Read the model definition and answer for the solid it produces. Units are mm, in the model's axes. Face numbers are marked on the shaded views. A direction names the side the tool comes from. Give positions to 0.01 mm unless a question says otherwise; leave off trailing zeros. Write each loop counter-clockwise with the first axis right and the second up, starting at its lowest first coordinate (ties: lowest second). Pieces come first, ordered by that corner, then holes.
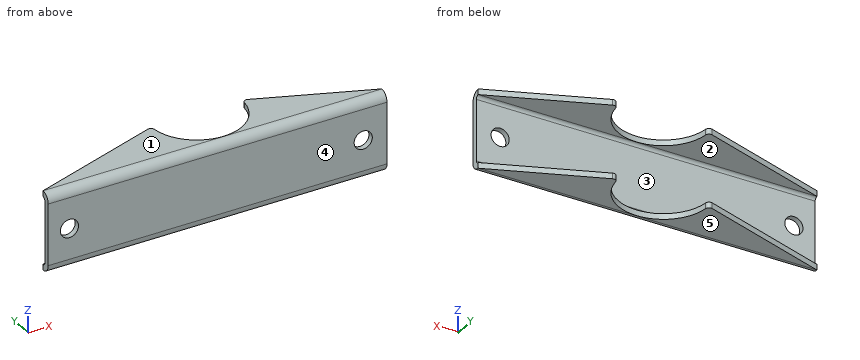
```python
from build123d import *

# Parameters (mm, degrees)
SKETCH1_W                      = 95.25
SKETCH1_H                      = 19.05
BASE_FLANGE1_DEPTH             = 1.5875
EDGE_FLANGE1_STRIP_W           = 8.128
EDGE_FLANGE1_STRIP_H           = 1.5875
EDGE_FLANGE1_STRIP_CUT_DEPTH   = 95.25
EDGE_FLANGE1_STRIP_2_W         = 8.128
EDGE_FLANGE1_STRIP_2_H         = 1.5875
EDGE_FLANGE1_STRIP_CUT_2_DEPTH = 95.25
EDGE_FLANGE1_DEPTH             = 95.25
EDGE_FLANGE1_BEND_DEPTH        = 95.25
CUT_EXTRUDE1_DEPTH             = 55.299926393
CUT_EXTRUDE1_DEPTH_BACK        = 55.299926393
HOLE1_START                    = -1.5875
HOLE1_OUTLINE_R                = 2.5527
HOLE1_DEPTH                    = 1.5875
FILLET1_R                      = 1


# Read off the part's stored shape, not the designer's step: Hole1
# Sheet-metal steps are written as plain solids
with BuildPart() as part:
    # Sketch1 → Base-Flange1 (new body)
    with BuildSketch(Plane(origin=(0, 0, 0), x_dir=(1, 0, 0), z_dir=(0, 1, 0))):
        Rectangle(SKETCH1_W, SKETCH1_H)
    extrude(amount=-BASE_FLANGE1_DEPTH)

    # Edge-Flange1 strip (across the edge) → Edge-Flange1 strip cut (cut)
    with BuildSketch(Plane(origin=(-47.625, 0, 9.525), x_dir=(0, 0, -1), z_dir=(1, 0, 0))):
        with Locations((-3.175, -0.79375)):
            Rectangle(EDGE_FLANGE1_STRIP_W, EDGE_FLANGE1_STRIP_H)
    extrude(amount=EDGE_FLANGE1_STRIP_CUT_DEPTH, mode=Mode.SUBTRACT)

    # Edge-Flange1 strip 2 (across the edge) → Edge-Flange1 strip cut 2 (cut)
    with BuildSketch(Plane(origin=(47.625, 0, -9.525), x_dir=(0, 0, 1), z_dir=(-1, 0, 0))):
        with Locations((-3.175, -0.79375)):
            Rectangle(EDGE_FLANGE1_STRIP_2_W, EDGE_FLANGE1_STRIP_2_H)
    extrude(amount=EDGE_FLANGE1_STRIP_CUT_2_DEPTH, mode=Mode.SUBTRACT)

    # Edge-Flange1 section (across the edge) → Edge-Flange1 (add)
    with BuildSketch(Plane(origin=(-47.625, 0, 9.525), x_dir=(0, 0, -1), z_dir=(1, 0, 0))):
        with BuildLine():
            Line((-1.5875, 0.889), (-1.5875, 13.6525))
            Line((-1.5875, 13.6525), (0, 13.6525))
            Line((0, 13.6525), (0, 0.889))
            ThreePointArc((0, 0.889), (0.260382072, 0.260382072), (0.889, 0))
            Line((0.889, 0), (0.889, -1.5875))
            ThreePointArc((0.889, -1.5875), (-0.862149944, -0.862149944), (-1.5875, 0.889))
        make_face()
    extrude(amount=EDGE_FLANGE1_DEPTH)

    # Edge-Flange1 section 2 (across the edge) → Edge-Flange1 bend (add)
    with BuildSketch(Plane(origin=(47.625, 0, -9.525), x_dir=(0, 0, 1), z_dir=(-1, 0, 0))):
        with BuildLine():
            Line((-1.5875, 0.889), (-1.5875, 13.6525))
            Line((-1.5875, 13.6525), (0, 13.6525))
            Line((0, 13.6525), (0, 0.889))
            ThreePointArc((0, 0.889), (0.260382072, 0.260382072), (0.889, 0))
            Line((0.889, 0), (0.889, -1.5875))
            ThreePointArc((0.889, -1.5875), (-0.862149944, -0.862149944), (-1.5875, 0.889))
        make_face()
    extrude(amount=EDGE_FLANGE1_BEND_DEPTH)

    # Sketch12 → Cut-Extrude1 (cut, two sides: drawn at the far end of the back side and taken through both)
    with BuildSketch(Plane.XY.offset(11.1125).offset(-CUT_EXTRUDE1_DEPTH_BACK)):
        with BuildLine():
            Line((15.847398271, 13.6525), (-9.552601729, 13.6525))
            ThreePointArc((-9.552601729, 13.6525), (3.147398271, 0.9525), (15.847398271, 13.6525))
        make_face()
        Polygon((-47.625, 0.889), (-9.552601729, 13.6525), (-47.625, 13.6525), align=None)
        Polygon((47.625, 13.6525), (15.847398271, 13.6525), (47.625, 0.889), align=None)
    extrude(amount=CUT_EXTRUDE1_DEPTH + CUT_EXTRUDE1_DEPTH_BACK, mode=Mode.SUBTRACT)

    # Hole1 outline → Hole1 (cut)
    with BuildSketch(Plane(origin=(0, 0, 0), x_dir=(1, 0, 0), z_dir=(0, 1, 0)).offset(HOLE1_START)):
        with Locations((40.940976195, 0)):
            Circle(HOLE1_OUTLINE_R)
        with Locations((-41.656, 0)):
            Circle(HOLE1_OUTLINE_R)
    extrude(amount=HOLE1_DEPTH, mode=Mode.SUBTRACT)

    # Fillet1
    fillet1_edges = [part.edges().sort_by_distance(p)[0] for p in [
        (-9.552601729, 13.6525, -10.31875),
        (15.847398271, 13.6525, 10.31875),
        (15.847398271, 13.6525, -10.31875),
        (-9.552601729, 13.6525, 10.31875),
    ]]
    fillet(fillet1_edges, radius=FILLET1_R)


solid = part.part
```
Item 1: This flat-tipped pin is pushed along its axis until it touches: pin 1 Ø5 at (x, z) = (6, -1) entering from +Y. Where does it stop, or does it pass through?
Result set:
pin 1: stops at y = 0
Item 2: Section A-A (z = 0) is taken. Write down the section's boundary in (x, y) (1 decimal), and give its area (3 significant figures).
Result set:
outline: (-47.6, -1.6) - (-44.2, -1.6) - (-44.2, 0) - (-47.6, 0) - close; (-39.1, -1.6) - (38.4, -1.6) - (38.4, 0) - (-39.1, 0) - close; (43.5, -1.6) - (47.6, -1.6) - (47.6, 0) - (43.5, 0) - close
area: 135 mm2
Item 3: Determine the mould class of the marked faces 3, 4 and 5 for opening direction Z: pulls with the +Z half, pulls with the -Z half, needs draft (parallel to the pull), parting line crosses it, or undercut.
Result set:
face 3: undercut
face 4: needs draft
face 5: pulls with the -Z half
Item 4: Section C-C (x = -35.5) is taken. Write down the section's boundary in (y, z) (1 decimal), and give its area (3 significant figures).
Result set:
outline: (-1.6, -8.6) arc R2.5 ccw to (0.9, -11.1) - (5, -11.1) - (5, -9.5) - (0.9, -9.5) arc R0.9 cw to (0, -8.6) - (0, 8.6) arc R0.9 cw to (0.9, 9.5) - (5, 9.5) - (5, 11.1) - (0.9, 11.1) arc R2.5 ccw to (-1.6, 8.6) - close
area: 48.7 mm2
Item 5: Which of the six approach directions +Z, -Z, +X, -X, +Y, -Y give full straight-line access (tool end or side, diameter ignored) to the marked faces 1 and 2?
Result set:
face 1: +Z, +X, -X, +Y, -Y
face 2: +X, -X, +Y
Item 6: Section D-D (y = 3.5) is taken. Write down the section's boundary in (x, z) (1 decimal).
Result set:
outline: (-39.8, -11.1) - (-4.5, -11.1) - (-4.5, -9.5) - (-39.8, -9.5) - close; (-39.8, 9.5) - (-4.5, 9.5) - (-4.5, 11.1) - (-39.8, 11.1) - close; (10.8, -11.1) - (41.1, -11.1) - (41.1, -9.5) - (10.8, -9.5) - close; (10.8, 9.5) - (41.1, 9.5) - (41.1, 11.1) - (10.8, 11.1) - close
Item 7: Section B-B (y = 11.5) is taken. Write down the section's boundary in (x, z) (1 decimal), and give its area (3 significant figures).
Result set:
outline: (-16, -11.1) - (-9.4, -11.1) - (-9.4, -9.5) - (-16, -9.5) - close; (-16, 9.5) - (-9.4, 9.5) - (-9.4, 11.1) - (-16, 11.1) - close; (15.7, -11.1) - (21.2, -11.1) - (21.2, -9.5) - (15.7, -9.5) - close; (15.7, 9.5) - (21.2, 9.5) - (21.2, 11.1) - (15.7, 11.1) - close
area: 38.6 mm2
Item 8: Find the intervals of material crossed by line 1 along X through (y, z) = (-1.1, 0) (3 decimals); line 2 along Z through (x, y) = (-26, 2.25) (1 decimal); line 3 along Y through (x, z) = (-33, 4.5), in increasing order.
Result set:
line 1: x = -47.625 to -44.209, -39.103 to 38.388, 43.494 to 47.625
line 2: z = -11.1 to -9.5, 9.5 to 11.1
line 3: y = -1.59 to 0
